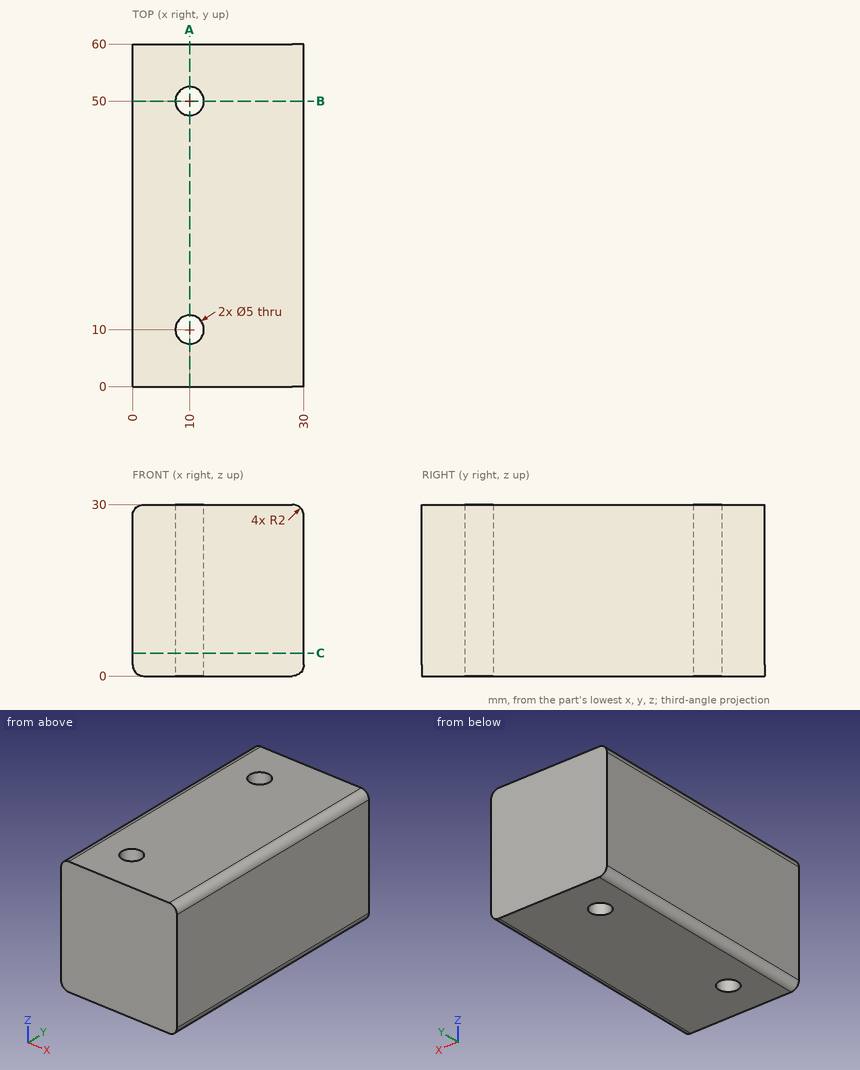
Part print with two shaded views. Sizes in mm from the minimum x, y, z corner. Give positions to 0.01 mm unless a question says otherwise; leave off trailing zeros. Order: outer loops, then holes, each group sorted by start corner. A loop starts at its lowest first (then second) coordinate and runs counter-clockwise, first axis right, second up.
1) Saw through at A-A, the plane x = 10. Write the cut outline in (y, z).
2) Wall check: probe 1 along Y at (x, z) = (10, 14); probe 2 along Y at (x, z) = (8.75, 6.25); probe 3 along X at (y, z) = (9, 5). Give the ranges that are in metal, low to high.
3) Saw through at B-B, the plane y = 50. Write the cut outline in (x, z), then the cut area to 3 significant figures.
4) Saw through at C-C, the plane z = 4. Write the cut outline in (x, y), then the cut area to 3 significant figures.
Computed:
1. outline: (0, 0) - (7.5, 0) - (7.5, 30) - (0, 30) - close; (12.5, 0) - (47.5, 0) - (47.5, 30) - (12.5, 30) - close; (52.5, 0) - (60, 0) - (60, 30) - (52.5, 30) - close
2. probe 1: y = 0 to 7.5, 12.5 to 47.5, 52.5 to 60
2. probe 2: y = 0 to 7.83, 12.17 to 47.83, 52.17 to 60
2. probe 3: x = 0 to 7.71, 12.29 to 30
3. outline: (0, 2) arc R2 ccw to (2, 0) - (7.5, 0) - (7.5, 30) - (2, 30) arc R2 ccw to (0, 28) - close; (12.5, 0) - (28, 0) arc R2 ccw to (30, 2) - (30, 28) arc R2 ccw to (28, 30) - (12.5, 30) - close
3. area: 747 mm2
4. outline: (0, 0) - (30, 0) - (30, 60) - (0, 60) - close; hole circle Ø5 at (10, 10); hole circle Ø5 at (10, 50)
4. area: 1,760 mm2
